Could you check a few things on this model? Use its own coordinates, in mm. Give positions to 0.01 mm unless a question says otherwise; leave off trailing zeros. Loops run counter-clockwise (first coordinate to the right, second up) from the corner with the lowest first, then second, coordinate; pieces in that order, holes last. Notation, with made-up numbers: M 60.25,64.25 L 79.25,64.25 A15 ccw 79.25,87.25 Z; hole C 61,75 d2. An arc over 180 degrees is marked long. Use CSV: the item, a comma, the result in double quotes.
```python
from build123d import *

# Parameters (mm, degrees)
SKETCH1_W           = 3
SKETCH1_H           = 30
SKETCH1_W_2         = 15.25
SKETCH1_H_2         = 3
BOSS_EXTRUDE1_DEPTH = 3


with BuildPart() as part:
    # Sketch1 → Boss-Extrude1 (new body)
    with BuildSketch(Plane(origin=(0, 0, 0), x_dir=(1, 0, 0), z_dir=(0, 1, 0))):
        Polygon((-95, 15), (-98, 15), (-98, -15), (-95, -15), (-95, -42), (-73.5, -42), (-73.5, -45), (-52.5, -45), (-52.5, -42), (-31.5, -42), (-31.5, -45), (-10.5, -45), (-10.5, -42), (10.5, -42), (10.5, -45), (31.5, -45), (31.5, -42), (52.5, -42), (52.5, -45), (73.5, -45), (73.5, -42), (95, -42), (95, -15), (98, -15), (98, 15), (95, 15), (95, 42), (73.5, 42), (73.5, 45), (52.5, 45), (52.5, 42), (31.5, 42), (31.5, 45), (10.5, 45), (10.5, 42), (-10.5, 42), (-10.5, 45), (-31.5, 45), (-31.5, 42), (-52.5, 42), (-52.5, 45), (-73.5, 45), (-73.5, 42), (-95, 42), align=None)
        Rectangle(SKETCH1_W, SKETCH1_H, mode=Mode.SUBTRACT)
        with Locations((48.25, 0)):
            Rectangle(SKETCH1_W, SKETCH1_H, mode=Mode.SUBTRACT)
        with Locations((72.375, 0)):
            Rectangle(SKETCH1_W_2, SKETCH1_H_2, mode=Mode.SUBTRACT)
        with Locations((-48.25, 0)):
            Rectangle(SKETCH1_W, SKETCH1_H, mode=Mode.SUBTRACT)
        with Locations((-24.125, 0)):
            Rectangle(SKETCH1_W_2, SKETCH1_H_2, mode=Mode.SUBTRACT)
        with Locations((24.125, 0)):
            Rectangle(SKETCH1_W_2, SKETCH1_H_2, mode=Mode.SUBTRACT)
    extrude(amount=BOSS_EXTRUDE1_DEPTH)


solid = part.part
```
1. I want a section at C-C, the plane x = -84. List the corners of the cut face in (y, z) for me, then the cut area to 3 significant figures.
Outcome:
outline,"M 0,-42 L 3,-42 L 3,42 L 0,42 Z"
area,"252 mm2"
2. Please list where these lines run through material, in increasing order: line 1 (X direction, y = 1.55, z = -13.5); line 2 (Z direction, x = 74, y = 0.55); line 3 (Z direction, x = 68, y = 2.35).
Outcome:
line 1,"-98 to -49.75, -46.75 to -1.5, 1.5 to 46.75, 49.75 to 98"
line 2,"-42 to -1.5, 1.5 to 42"
line 3,"-45 to -1.5, 1.5 to 45"
3. I want a section at B-B, the plane y = 1.4. Give the number of separate pieces and of enclosed holes in the cut face, then the cut area to 3 significant figures.
Outcome:
separate pieces,"1"
enclosed holes,"6"
area,"16,200 mm2"
4. I want a section at D-D, the plane z = -19. List the corners of the cut face in (x, y) for me, then the cut area to 3 significant figures.
Outcome:
outline,"M -95,0 L 95,0 L 95,3 L -95,3 Z"
area,"570 mm2"
5. I'm going to push flat-ended pins straight in: pin 1 Ø1.5 at (x, y) = (-39, 1) entering from +Z; pin 2 Ø0.9 at (y, z) = (1.5, -44) entering from -X; pin 3 Ø1.5 at (x, y) = (-37, 1) entering from -Z. Where does each tip first touch, or does it pass through?
Outcome:
pin 1,"z = 42"
pin 2,"x = -73.5"
pin 3,"z = -42"
6. I want a section at A-A, the plane z = 12.5. List the corners of the cut face in (x, y) for me.
Outcome:
outline,"M -98,0 L -49.75,0 L -49.75,3 L -98,3 Z; M -46.75,0 L -1.5,0 L -1.5,3 L -46.75,3 Z; M 1.5,0 L 46.75,0 L 46.75,3 L 1.5,3 Z; M 49.75,0 L 98,0 L 98,3 L 49.75,3 Z"
